Check sheet for the modelled part. Datum: model origin and axes. Units: mm. A direction names the side the tool comes from. Round coordinates to 2 decimals unless told otherwise and drop trailing zeros. Write each loop counter-clockwise with the first axis right and the second up, starting at its lowest first coordinate (ties: lowest second). Pieces come first, ordered by that corner, then holes. Notation, with made-up numbers: (0.5, 12.25) - (26.5, 12.25) arc R13 cw to (26.5, 34.25) - close; hole circle Ø8 at (80, 5.5). An arc over 180 degrees is marked (long way). Use one line per item in the form item = value. Start each with the question number.
1) Scan lines: probe 1 along X at (y, z) = (22, -11); probe 2 along X at (y, z) = (28, -11); probe 3 along Z at (x, y) = (12.5, 48.5). Record each from-to range of solid material in increasing order.
2) Section check A-A (y = 10). Record the boundary of the cut face in (x, z).
3) Draft check along Z on faces 4 (the face through (-8.5, 78.2, -6.1)), 5 (the face through (17.99, 40.56, 18.15)), 6 (the face through (-1.73, 17.81, -18.46)). Enter one of: +Z half, -Z half, draft (parallel to the pull), parting line (faces both ways), or undercut.
4) Section check C-C (x = 0). Record the boundary of the cut face in (y, z), then the cut area to 3 significant figures.
5) Section check B-B (z = 0). Record the boundary of the cut face in (x, y), then the cut area to 3 significant figures.
6) Section check D-D (y = 69). Record the boundary of the cut face in (x, z).
7) Set-up check for faces 1 (the face through (16, 16.6, 0.1)), 2 (the face through (-8.5, 78.2, 15.9)), 3 (the face through (-16, 23.4, 0.1)): record each of +Z, -Z, +X, -X, +Y, -Y from which the full face is reachable in a straight line by a thin tool's end or side.
8) Gauge pin test, flat ends, axial feed: P1, Ø13, axis at x = 1, y = 9, coming from the -Z side; P2, Ø5, axis at y = 57, z = 14.5, coming from the +X side; P3, Ø7, axis at x = 0, y = 10, coming from the +Z side. Record the tip position at first contact, or that the pin passes through.
from build123d import *

# Parameters (mm, degrees)
SKETCH1_W                                        = 42
SKETCH1_H                                        = 42
BOSS_EXTRUDE1_DEPTH                              = 80
SKETCH2_R                                        = 6
CUT_EXTRUDE1_DEPTH                               = 93.763139231
SKETCH3_R                                        = 6
CUT_EXTRUDE2_DEPTH                               = 93.763139231
SKETCH4_R                                        = 3
CUT_EXTRUDE3_DEPTH                               = 93.763139231
SKETCH5_R                                        = 8
CUT_EXTRUDE4_DEPTH                               = 5
CUT_EXTRUDE5_START                               = -5
SKETCH6_R                                        = 8
CUT_EXTRUDE5_DEPTH                               = 5
SKETCH7_R                                        = 3
CUT_EXTRUDE6_DEPTH                               = 93.763139231
SKETCH8_R                                        = 8
CUT_EXTRUDE7_DEPTH                               = 5
CUT_EXTRUDE8_START                               = -5
SKETCH9_R                                        = 8
CUT_EXTRUDE8_DEPTH                               = 5
FILLET1_R                                        = 10
CBORE_FOR_M5_PAN_HEAD_MACHINE_SCREW1_D           = 5.3
CBORE_FOR_M5_PAN_HEAD_MACHINE_SCREW1_CBORE_D     = 11
CBORE_FOR_M5_PAN_HEAD_MACHINE_SCREW1_CBORE_DEPTH = 3.7


with BuildPart() as part:
    # Sketch1 → Boss-Extrude1 (new body)
    with BuildSketch(Plane(origin=(0, 0, 0), x_dir=(1, 0, 0), z_dir=(0, 1, 0))):
        Rectangle(SKETCH1_W, SKETCH1_H)
    extrude(amount=BOSS_EXTRUDE1_DEPTH)

    # Sketch2 → Cut-Extrude1 (cut, through all)
    with BuildSketch(Plane.XY.offset(21)):
        with Locations((0, 32)):
            Circle(SKETCH2_R)
    extrude(amount=-CUT_EXTRUDE1_DEPTH, mode=Mode.SUBTRACT)

    # Sketch3 → Cut-Extrude2 (cut, through all)
    with BuildSketch(Plane(origin=(21, 0, 0), x_dir=(0, 0, -1), z_dir=(1, 0, 0))):
        with Locations((0, 47)):
            Circle(SKETCH3_R)
    extrude(amount=-CUT_EXTRUDE2_DEPTH, mode=Mode.SUBTRACT)

    # Sketch4 → Cut-Extrude3 (cut, through all)
    with BuildSketch(Plane.XY.offset(21)):
        with Locations((0, 10)):
            Circle(SKETCH4_R)
    extrude(amount=-CUT_EXTRUDE3_DEPTH, mode=Mode.SUBTRACT)

    # Sketch5 → Cut-Extrude4 (cut)
    with BuildSketch(Plane.XY.offset(21)):
        with Locations((0, 10)):
            Circle(SKETCH5_R)
    extrude(amount=-CUT_EXTRUDE4_DEPTH, mode=Mode.SUBTRACT)

    # Sketch6 → Cut-Extrude5 (cut)
    with BuildSketch(Plane(origin=(0, 0, -21), x_dir=(-1, 0, 0), z_dir=(0, 0, -1)).offset(CUT_EXTRUDE5_START)):
        with Locations(Location((0, 10, 0), (0, 0, 180))):
            Circle(SKETCH6_R)
    extrude(amount=CUT_EXTRUDE5_DEPTH, mode=Mode.SUBTRACT)

    # Sketch7 → Cut-Extrude6 (cut, through all)
    with BuildSketch(Plane(origin=(21, 0, 0), x_dir=(0, 0, -1), z_dir=(1, 0, 0))):
        with Locations((0, 20)):
            Circle(SKETCH7_R)
    extrude(amount=-CUT_EXTRUDE6_DEPTH, mode=Mode.SUBTRACT)

    # Sketch8 → Cut-Extrude7 (cut)
    with BuildSketch(Plane(origin=(21, 0, 0), x_dir=(0, 0, -1), z_dir=(1, 0, 0))):
        with Locations((0, 20)):
            Circle(SKETCH8_R)
    extrude(amount=-CUT_EXTRUDE7_DEPTH, mode=Mode.SUBTRACT)

    # Sketch9 → Cut-Extrude8 (cut)
    with BuildSketch(Plane.ZY.offset(21).offset(CUT_EXTRUDE8_START)):
        with Locations(Location((0, 20, 0), (0, 0, 180))):
            Circle(SKETCH9_R)
    extrude(amount=CUT_EXTRUDE8_DEPTH, mode=Mode.SUBTRACT)

    # Fillet1
    fillet1_edges = [part.edges().sort_by_distance(p)[0] for p in [
        (21, 40, 21),
        (-21, 40, 21),
        (-21, 40, -21),
        (21, 40, -21),
    ]]
    fillet(fillet1_edges, radius=FILLET1_R)

    # CBORE for M5 Pan Head Machine Screw1 (through all)
    with Locations(Plane(origin=(0, 80, 0), x_dir=(1, 0, 0), z_dir=(0, 1, 0))):
        with Locations((-11, 11), (11, 11), (11, -11), (-11, -11)):
            CounterBoreHole(CBORE_FOR_M5_PAN_HEAD_MACHINE_SCREW1_D / 2, CBORE_FOR_M5_PAN_HEAD_MACHINE_SCREW1_CBORE_D / 2, CBORE_FOR_M5_PAN_HEAD_MACHINE_SCREW1_CBORE_DEPTH)


solid = part.part
Results are:
q1.probe_1 = -21 to -13.65, -8.35 to 8.35, 13.65 to 21
q1.probe_2 = -21 to -13.65, -8.35 to -4.47, 4.47 to 8.35, 13.65 to 21
q1.probe_3 = -20.89 to -13.18, -8.82 to -5.81, 5.81 to 8.82, 13.18 to 20.89
q2.outline = (-21, -11) arc R10 ccw to (-11, -21) - (-8, -21) - (-8, -16) - (-3, -16) - (-3, 16) - (-8, 16) - (-8, 21) - (-11, 21) arc R10 ccw to (-21, 11) - close; (3, -16) - (8, -16) - (8, -21) - (11, -21) arc R10 ccw to (21, -11) - (21, 11) arc R10 ccw to (11, 21) - (8, 21) - (8, 16) - (3, 16) - close; hole circle Ø5.3 at (-11, -11); hole circle Ø5.3 at (-11, 11); hole circle Ø5.3 at (11, -11); hole circle Ø5.3 at (11, 11)
q3.face_4 = undercut
q3.face_5 = +Z half
q3.face_6 = draft
q4.outline = (0, -21) - (2, -21) - (2, -16) - (7, -16) - (7, 16) - (2, 16) - (2, 21) - (0, 21) - close; (13, -16) - (18, -16) - (18, -21) - (26, -21) - (26, 21) - (18, 21) - (18, 16) - (13, 16) - close; (38, -21) - (80, -21) - (80, 21) - (38, 21) - close; hole circle Ø6 at (20, 0); hole circle Ø12 at (47, 0)
q4.area = 2,360 mm²
q5.outline = (-21, 0) - (21, 0) - (21, 12) - (16, 12) - (16, 17) - (-16, 17) - (-16, 12) - (-21, 12) - close; (-21, 28) - (-16, 28) - (-16, 23) - (16, 23) - (16, 28) - (21, 28) - (21, 41) - (-21, 41) - close; (-21, 53) - (21, 53) - (21, 80) - (-21, 80) - close; hole circle Ø12 at (0, 32); hole circle Ø6 at (0, 10)
q5.area = 2,360 mm²
q6.outline = (-21, -11) arc R10 ccw to (-11, -21) - (11, -21) arc R10 ccw to (21, -11) - (21, 11) arc R10 ccw to (11, 21) - (-11, 21) arc R10 ccw to (-21, 11) - close; hole circle Ø5.3 at (-11, -11); hole circle Ø5.3 at (-11, 11); hole circle Ø5.3 at (11, -11); hole circle Ø5.3 at (11, 11)
q7.face_1 = +X
q7.face_2 = +Y
q7.face_3 = -X
q8.P1 = -16
q8.P2 = 20.95
q8.P3 = 16
